Input: dimensioned drawing with shaded views. Units: mm. Origin: part minimum x, y, z. Give positions to 0.01 mm unless a question says otherwise; leave off trailing zeros. Write each loop counter-clockwise with the first axis right and the second up, starting at its lowest first coordinate (ties: lowest second). Pieces come first, ordered by that corner, then holes.
Q1. Line query: line 1 (Y direction, x = 70, z = 0.75); line 2 (Y direction, x = 106, z = 5); line 3 (X direction, y = 22.5, z = 4.25). Output: solid intervals per line, ascending.
Q2. Section C-C (z = 8). Return the cut outline in (x, y).
Q3. Section B-B (y = 17.5). Return the cut outline in (x, z).
Q4. Pin query (flat end, axial travel): pin 1 Ø6 at (y, z) = (39.5, 5.5) entering from -X; pin 2 Ø4 at (y, z) = (71.5, 6) entering from -X. Return the tip coordinate at first contact, or that it passes through.
Q5. Section A-A (x = 36). Return the cut outline in (y, z), plus the area to 3 significant figures.
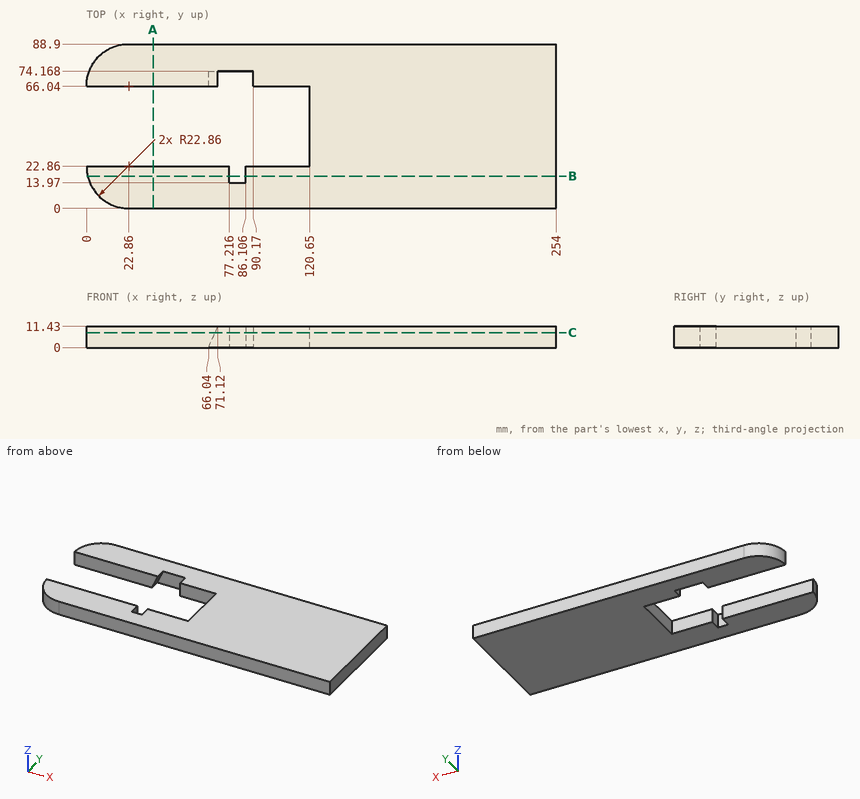
Computed:
1. line 1: y = 0 to 22.86, 74.17 to 88.9
1. line 2: y = 0 to 22.86, 66.04 to 88.9
1. line 3: x = 0 to 77.22, 86.11 to 254
2. outline: (0, 22.86) arc R22.86 ccw to (22.86, 0) - (254, 0) - (254, 88.9) - (22.86, 88.9) arc R22.86 ccw to (0, 66.04) - (69.6, 66.04) - (69.6, 74.17) - (90.17, 74.17) - (90.17, 66.04) - (120.65, 66.04) - (120.65, 22.86) - (86.11, 22.86) - (86.11, 13.97) - (77.22, 13.97) - (77.22, 22.86) - close
3. outline: (0.64, 0) - (77.22, 0) - (77.22, 11.43) - (0.64, 11.43) - close; (86.11, 0) - (254, 0) - (254, 11.43) - (86.11, 11.43) - close
4. pin 1: stops at x = 120.65
4. pin 2: stops at x = 0.26
5. outline: (0, 0) - (22.86, 0) - (22.86, 11.43) - (0, 11.43) - close; (66.04, 0) - (88.9, 0) - (88.9, 11.43) - (66.04, 11.43) - close
5. area: 523 mm2
